Autodesk Inventor part; units mm, degrees
ref_plane "YZ Plane" through (0, 0, 0) normal (1, 0, 0) x (0, 1, 0)
ref_plane "XZ Plane" through (0, 0, 0) normal (0, 1, 0) x (-1, 0, 0)
ref_plane "XY Plane" through (0, 0, 0) normal (0, 0, 1) x (1, 0, 0)
sketch "Sketch1" plane through (0, 0, 0) normal (0, 0, 1) x (1, 0, 0)
  circle A0 centre (0, 0) radius 6.35
  dimension "d0" = 12.7
extrude "Extrusion1" add sketch "Sketch1" along normal blind 1.5875
sketch "Sketch2" plane through (0, 0, 1.5875) normal (0, 0, 1) x (1, 0, 0)
  circle A0 centre (0, 0) radius 6.35
  circle A1 centre (0, 0) radius 3.9688
  dimension "d3" = 7.9375
extrude "Extrusion2" add sketch "Sketch2" along normal blind 24.1745 contours A1
fillet "Fillet1" radius 3.175 1 edges at (-3.9688, 0, 1.5875)
sketch "Sketch3" plane through (0, 0, 25.762) normal (0, 0, 1) x (1, 0, 0)
  circle A0 centre (0, 0) radius 3.9687
hole "Hole1" at (0, 0, 25.762) direction (0, 0, -1) diameter 4.9784 end through all
properties part number "Pneumatic Standoff Curved" material "Aluminum 6061"
Part model, mm, in its own coordinate system. A direction names the side the tool comes from. Round coordinates to 2 decimals unless told otherwise and drop trailing zeros. Order: outer loops, then holes, each group sorted by start corner. A loop starts at its lowest first (then second) coordinate and runs counter-clockwise, first axis right, second up. Notation, with made-up numbers: M 31,46.5 L 78,46.5 A12 ccw 78,61.5 Z; hole C 67.5,7.5 d5. An arc over 180 degrees is marked long. Answer in a Markdown table with one row per item. Add a question column.
Q1. Cut at C-C on z = 5.75. Give the cut face in (x, y).
Q2. Pin check, flat tips, straight feed: pin 1 (2 mm diameter, centred on y = -2.5, z = 16.5, fed in from -X); pin 2 (2 mm diameter, centred on y = 1.5, z = 22, fed in from +X); pin 3 (1.5 mm diameter, centred on x = -5, z = 16, fed in from +Y); pin 4 (3 mm diameter, centred on y = -3, z = 8.5, fed in from +X). Stop position of each tip, or through.
Q3. 3-axis set-ups, long thin cutter, end or side, ignore diameter. For faces 4 (the face through (3, 0, 0)), 5 (the face through (3.666, 1.52, 15.064)): which of +Z, -Z, +X, -X, +Y, -Y reach the whole face in a straight line?
Q4. Mould opens along X. For faces 1 (the face through (-1.38, 6.2, 0.78)), 2 (the face through (-0.748, -2.374, 12.701)), 3 (the face through (2, 2, 25.762)) say: +X half, -X half, draft (parallel to the pull), parting line (faces both ways), or undercut.
Q5. Wall check: L1, parallel to Y at x = 0, z = 13.75; L2, parallel to Y at x = -0.5, z = 6.25; L3, parallel to Z at x = 5, y = -1.5. Give the ranges that are in metal, low to high. Write a range as from..to.
Established:
| question | item | result |
|---|---|---|
| 1 | outline | C 0,0 d7.94; hole C 0,0 d4.98 |
| 2 | pin 1 | stops at x = -3.67 |
| 2 | pin 2 | stops at x = 3.94 |
| 2 | pin 3 | passes through |
| 2 | pin 4 | stops at x = 3.67 |
| 3 | face 4 | -Z, +X, -X, +Y, -Y |
| 3 | face 5 | +Z |
| 4 | face 1 | parting line |
| 4 | face 2 | undercut |
| 4 | face 3 | draft |
| 5 | L1 | y = -3.97..-2.49, 2.49..3.97 |
| 5 | L2 | y = -3.94..-2.44, 2.44..3.94 |
| 5 | L3 | z = 0..2.14 |
